CAD build for the part. Positions are in the model's coordinates, mm. Give positions to 0.01 mm unless a question says otherwise; leave off trailing zeros. Write each loop counter-clockwise with the first axis right and the second up, starting at its lowest first coordinate (ties: lowest second). Pieces come first, ordered by that corner, then holes. Notation, with made-up numbers: (-7.5, 73.5) - (19.5, 73.5) arc R22 cw to (19.5, 85.5) - close; hole circle Ø11 at (43, 53). An arc over 180 degrees is marked (long way). Answer as a JSON object with one key per item and string values.
from build123d import *

# Parameters (mm, degrees)
ESQUISSE1_W              = 203.2
ESQUISSE1_H              = 203.2
BOSS_EXTRU_1_DEPTH       = 6.35
ESQUISSE2_R              = 4
ENL_V_MAT_EXTRU_1_DEPTH  = 144.824345992
ENL_V_MAT_EXTRU_2_DEPTH  = 144.824345992
ENL_V_MAT_EXTRU_3_DEPTH  = 144.824345992
CONG_1_R                 = 5
ENL_V_MAT_EXTRU_5_DEPTH  = 144.824345992
ENL_V_MAT_EXTRU_6_DEPTH  = 144.824345992
ENL_V_MAT_EXTRU_7_DEPTH  = 144.824345992
ENL_V_MAT_EXTRU_8_DEPTH  = 144.824345992
ENL_V_MAT_EXTRU_9_DEPTH  = 144.824345992
ESQUISSE11_R             = 2.5
ENL_V_MAT_EXTRU_10_DEPTH = 144.824345992


with BuildPart() as part:
    # Esquisse1 → Boss.-Extru.1 (new body)
    with BuildSketch(Plane(origin=(0, 0, 0), x_dir=(1, 0, 0), z_dir=(0, 1, 0))):
        Rectangle(ESQUISSE1_W, ESQUISSE1_H)
    extrude(amount=BOSS_EXTRU_1_DEPTH)

    # Esquisse2 → Enlèv. mat.-Extru.1 (cut, through all)
    with BuildSketch(Plane(origin=(0, 6.35, 0), x_dir=(1, 0, 0), z_dir=(0, 1, 0))):
        with Locations(Location((-75, 65, 0), (0, 0, 270))):
            Circle(ESQUISSE2_R)
        with Locations(Location((75, 65, 0), (0, 0, 270))):
            Circle(ESQUISSE2_R)
        with Locations(Location((0, -65, 0), (0, 0, 270))):
            Circle(ESQUISSE2_R)
    extrude(amount=-ENL_V_MAT_EXTRU_1_DEPTH, mode=Mode.SUBTRACT)

    # Esquisse3 → Enlèv. mat.-Extru.2 (cut, through all)
    with BuildSketch(Plane(origin=(0, 6.35, 0), x_dir=(1, 0, 0), z_dir=(0, 1, 0))):
        Polygon((-17.05, 86.15), (-21.15, 82.05), (-21.15, 47.95), (-17.05, 43.85), (17.05, 43.85), (21.15, 47.95), (21.15, 82.05), (17.05, 86.15), align=None)
    extrude(amount=-ENL_V_MAT_EXTRU_2_DEPTH, mode=Mode.SUBTRACT)

    # Esquisse4 → Enlèv. mat.-Extru.3 (cut, through all)
    with BuildSketch(Plane(origin=(0, 6.35, 0), x_dir=(1, 0, 0), z_dir=(0, 1, 0))):
        Polygon((-49.6, -101.6), (-39.6, -101.6), (-39.6, 59), (-21.15, 59), (-21.15, 71), (-49.6, 71), align=None)
    extrude(amount=-ENL_V_MAT_EXTRU_3_DEPTH, mode=Mode.SUBTRACT)

    # Congé1
    cong_1_edges = [part.edges().sort_by_distance(p)[0] for p in [
        (-49.6, 3.175, -71),
        (-39.6, 3.175, -59),
    ]]
    fillet(cong_1_edges, radius=CONG_1_R)

    # Esquisse5 → Enlèv. mat.-Extru.5 (cut, through all)
    with BuildSketch(Plane(origin=(0, 6.35, 0), x_dir=(1, 0, 0), z_dir=(0, 1, 0))):
        Polygon((-28.852385868, 49.85), (-31.138692934, 45.89), (-35.711307066, 45.89), (-37.997614132, 49.85), (-35.711307066, 53.81), (-31.138692934, 53.81), align=None)
    extrude(amount=-ENL_V_MAT_EXTRU_5_DEPTH, mode=Mode.SUBTRACT)

    # Esquisse7 → Enlèv. mat.-Extru.6 (cut, through all)
    with BuildSketch(Plane(origin=(0, 6.35, 0), x_dir=(1, 0, 0), z_dir=(0, 1, 0))):
        Polygon((-31.138692934, 75.89), (-35.711307066, 75.89), (-37.997614132, 79.85), (-35.711307066, 83.81), (-31.138692934, 83.81), (-28.852385868, 79.85), align=None)
    extrude(amount=-ENL_V_MAT_EXTRU_6_DEPTH, mode=Mode.SUBTRACT)

    # Esquisse8 → Enlèv. mat.-Extru.7 (cut, through all)
    with BuildSketch(Plane(origin=(0, 6.35, 0), x_dir=(1, 0, 0), z_dir=(0, 1, 0))):
        Polygon((36.011307066, 45.89), (31.438692934, 45.89), (29.152385868, 49.85), (31.438692934, 53.81), (36.011307066, 53.81), (38.297614132, 49.85), align=None)
    extrude(amount=-ENL_V_MAT_EXTRU_7_DEPTH, mode=Mode.SUBTRACT)

    # Esquisse9 → Enlèv. mat.-Extru.8 (cut, through all)
    with BuildSketch(Plane(origin=(0, 6.35, 0), x_dir=(1, 0, 0), z_dir=(0, 1, 0))):
        Polygon((36.011307066, 75.89), (31.438692934, 75.89), (29.152385868, 79.85), (31.438692934, 83.81), (36.011307066, 83.81), (38.297614132, 79.85), align=None)
    extrude(amount=-ENL_V_MAT_EXTRU_8_DEPTH, mode=Mode.SUBTRACT)

    # Esquisse10 → Enlèv. mat.-Extru.9 (cut, through all)
    with BuildSketch(Plane(origin=(0, 6.35, 0), x_dir=(1, 0, 0), z_dir=(0, 1, 0))):
        Polygon((20.1610714, -74), (17.874764334, -70.04), (13.302150202, -70.04), (11.015843136, -74), (13.302150202, -77.96), (17.874764334, -77.96), align=None)
        Polygon((-20.1610714, -74), (-17.874764334, -77.96), (-13.302150202, -77.96), (-11.015843136, -74), (-13.302150202, -70.04), (-17.874764334, -70.04), align=None)
        Polygon((-4.572614132, -47), (-2.286307066, -50.96), (2.286307066, -50.96), (4.572614132, -47), (2.286307066, -43.04), (-2.286307066, -43.04), align=None)
        Polygon((-63.984156864, 56), (-61.697849798, 52.04), (-57.125235666, 52.04), (-54.8389286, 56), (-57.125235666, 59.96), (-61.697849798, 59.96), align=None)
        Polygon((-95.1610714, 56), (-92.874764334, 52.04), (-88.302150202, 52.04), (-86.015843136, 56), (-88.302150202, 59.96), (-92.874764334, 59.96), align=None)
        Polygon((-79.572614132, 83), (-77.286307066, 79.04), (-72.713692934, 79.04), (-70.427385868, 83), (-72.713692934, 86.96), (-77.286307066, 86.96), align=None)
        Polygon((54.8389286, 56), (57.125235666, 52.04), (61.697849798, 52.04), (63.984156864, 56), (61.697849798, 59.96), (57.125235666, 59.96), align=None)
        Polygon((95.1610714, 56), (92.874764334, 59.96), (88.302150202, 59.96), (86.015843136, 56), (88.302150202, 52.04), (92.874764334, 52.04), align=None)
        Polygon((70.427385868, 83), (72.713692934, 79.04), (77.286307066, 79.04), (79.572614132, 83), (77.286307066, 86.96), (72.713692934, 86.96), align=None)
    extrude(amount=-ENL_V_MAT_EXTRU_9_DEPTH, mode=Mode.SUBTRACT)

    # Esquisse11 → Enlèv. mat.-Extru.10 (cut, through all)
    with BuildSketch(Plane(origin=(0, 6.35, 0), x_dir=(1, 0, 0), z_dir=(0, 1, 0))):
        with Locations(Location((93.6, 93.6, 0), (0, 0, 270))):
            Circle(ESQUISSE11_R)
        with Locations(Location((-93.6, 93.6, 0), (0, 0, 270))):
            Circle(ESQUISSE11_R)
        with Locations(Location((-93.6, -93.6, 0), (0, 0, 270))):
            Circle(ESQUISSE11_R)
        with Locations(Location((93.6, -93.6, 0), (0, 0, 270))):
            Circle(ESQUISSE11_R)
    extrude(amount=-ENL_V_MAT_EXTRU_10_DEPTH, mode=Mode.SUBTRACT)


solid = part.part
(1) Saw through at D-D, the plane z = -93.6. Give the cut face in (x, y).
Answer key:
{"outline": "(-101.6, 0) - (-96.1, 0) - (-96.1, 6.35) - (-101.6, 6.35) - close; (-91.1, 0) - (91.1, 0) - (91.1, 6.35) - (-91.1, 6.35) - close; (96.1, 0) - (101.6, 0) - (101.6, 6.35) - (96.1, 6.35) - close"}
(2) Saw through at A-A, the plane z = 65. Give the cut face in (x, y), and give its area (3 significant figures).
Answer key:
{"outline": "(-101.6, 0) - (-49.6, 0) - (-49.6, 6.35) - (-101.6, 6.35) - close; (-39.6, 0) - (-4, 0) - (-4, 6.35) - (-39.6, 6.35) - close; (4, 0) - (101.6, 0) - (101.6, 6.35) - (4, 6.35) - close", "area": "1,180 mm²"}
(3) Probe L1, parallel to Z at x = 33, y = 1.5; L2, parallel to X at y = 3, z = -65; L3, parallel to X at y = 2.25, z = 93.6. List the from-to ranges inside material, lowest first. Write a range as [from, to].
Answer key:
{"L1": "z = [-101.6, -83.81], [-75.89, -53.81], [-45.89, 101.6]", "L2": "x = [-101.6, -79], [-71, -49.6], [21.15, 71], [79, 101.6]", "L3": "x = [-101.6, -96.1], [-91.1, -49.6], [-39.6, 91.1], [96.1, 101.6]"}
(4) Saw through at C-C, the plane y = 2.75. State how many separate pieces and enclosed holes the cut face has, and give its area (3 significant figures).
Answer key:
{"separate pieces": "1", "enclosed holes": "20", "area": "36,700 mm²"}
(5) Pull direction X, two halves, no side cores. Call faces 1 (the face through (0, 3, -43.85)), 2 (the face through (-101.6, 3, 1)), 3 (the face through (-1, 6.35, -1)): pulls with the +X half, pulls with the -X half, needs draft (parallel to the pull), parting line crosses it, or undercut.
Answer key:
{"face 1": "undercut", "face 2": "pulls with the -X half", "face 3": "needs draft"}
(6) Saw through at B-B, the plane z = -31. Give the cut face in (x, y), and give its area (3 significant figures).
Answer key:
{"outline": "(-101.6, 0) - (-49.6, 0) - (-49.6, 6.35) - (-101.6, 6.35) - close; (-39.6, 0) - (101.6, 0) - (101.6, 6.35) - (-39.6, 6.35) - close", "area": "1,230 mm²"}
(7) Flat gauge pins, fed straight in: P1, Ø6.5, axis at x = -93.6, z = 93.6, coming from the -Y side; P2, Ø6.5, axis at x = 0, z = 65, coming from the -Y side. Where does each tip first touch, or does it go through?
Answer key:
{"P1": "stops at y = 0", "P2": "passes through"}
